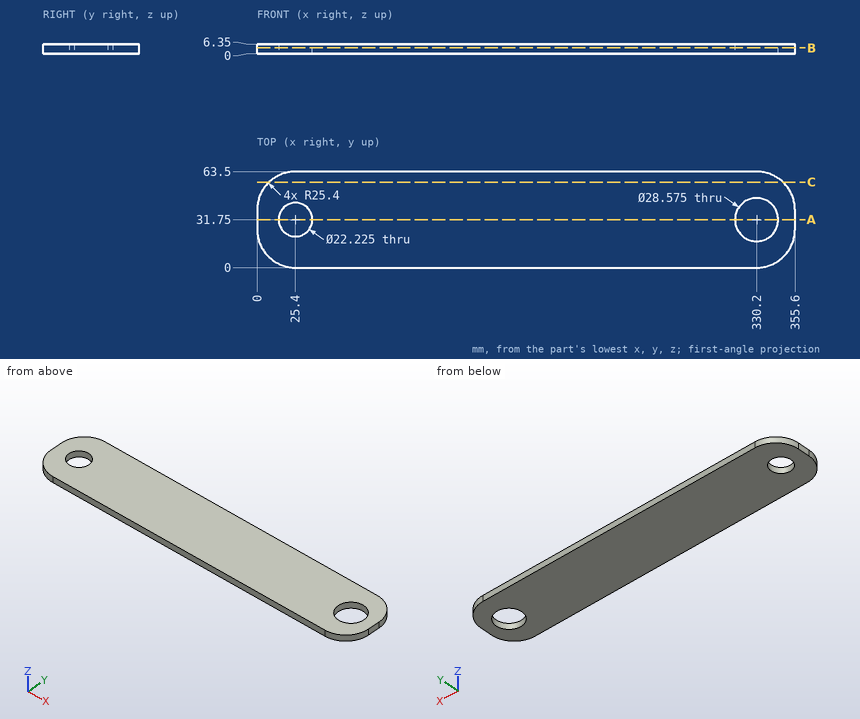
Study the drawing (mm; zero at the part's minimum x, y, z) and answer. Round coordinates to 2 decimals unless told otherwise and drop trailing zeros. Loops run counter-clockwise (first coordinate to the right, second up) from the corner with the lowest first, then second, coordinate; pieces in that order, holes last. Notation, with made-up numbers: (89, 68) -> (113, 68) arc R23 ccw to (113, 85) -> close; hole circle Ø1 at (-10, -34). An arc over 180 degrees is marked (long way). Write each question's results on one line, items separated by ' | '. Start each with the question number.
1. Section B-B (z = 3.75) is taken. State how many separate pieces and enclosed holes the cut face has, plus the area to 3 significant figures.
2. Section A-A (y = 31.75) is taken. Determine the outline of the cut face in (x, z).
3. Section C-C (y = 56.5) is taken. Determine the outline of the cut face in (x, z).
4. Find the intervals of material crossed by probe 1 along X at (y, z) = (26, 4.5); probe 2 along Y at (x, z) = (341, 5.5); probe 3 along X at (y, z) = (15, 2.25), in increasing order. Write a range as from..to.
Evaluation:
1) separate pieces: 1 | enclosed holes: 2 | area: 21,000 mm2
2) outline: (0, 0) -> (14.29, 0) -> (14.29, 6.35) -> (0, 6.35) -> close; (36.51, 0) -> (315.91, 0) -> (315.91, 6.35) -> (36.51, 6.35) -> close; (344.49, 0) -> (355.6, 0) -> (355.6, 6.35) -> (344.49, 6.35) -> close
3) outline: (7.89, 0) -> (347.71, 0) -> (347.71, 6.35) -> (7.89, 6.35) -> close
4) probe 1: x = 0..15.89, 34.91..317.12, 343.28..355.6 | probe 2: y = 2.41..22.4, 41.1..61.09 | probe 3: x = 2.23..353.37
